Verification items for the finished model (mm, model axes). Face numbers are marked on the shaded views. A direction names the side the tool comes from. Give positions to 0.01 mm unless a question says otherwise; leave off trailing zeros. Write each loop counter-clockwise with the first axis right and the second up, starting at its lowest first coordinate (ties: lowest second). Pieces come first, ordered by that corner, then holes. Notation, with made-up numbers: M 12,-27 L 52,-27 A13 ccw 52,-4 Z; hole C 5,-39.5 d4. An arc over 180 degrees is marked long. Write item = value, one per line.
from build123d import *

# Parameters (mm, degrees)
F1_DEPTH = 4
F2_R     = 2
F2_R_2   = 3.5
F3_DEPTH = 25
F4_R     = 4.99999


# Not quite as in the source:
# - a fillet or chamfer is up to 0.001 mm smaller than in the source, because OpenCascade refuses the exact size


with BuildPart() as f1:
    # F0 (on Top) → F1 (new body)
    with BuildSketch(Plane.XY):
        Polygon((-5, 65), (-5, 0), (-30, 0), (-30, -14), (30, -14), (30, 0), (5, 0), (5, 65), align=None)
    extrude(amount=F1_DEPTH)

    # F2 (on face) → F3 (cut)
    with BuildSketch(Plane.XY.offset(4)):
        with Locations((-25, -7)):
            Circle(F2_R)
        with Locations((25, -7)):
            Circle(F2_R)
        with Locations((0, -7)):
            Circle(F2_R_2)
        with Locations((0, 61)):
            Circle(F2_R)
    extrude(amount=-F3_DEPTH, mode=Mode.SUBTRACT)

    # F4 (radius 5 in the source; OpenCascade refuses exactly that, so slightly less here)
    f4_edges = [f1.edges().sort_by_distance(p)[0] for p in [
        (-30, -14, 2),
        (-30, 0, 2),
        (30, -14, 2),
        (30, 0, 2),
        (5, 65, 2),
        (-5, 65, 2),
    ]]
    fillet(f4_edges, radius=F4_R)


solid = f1.part
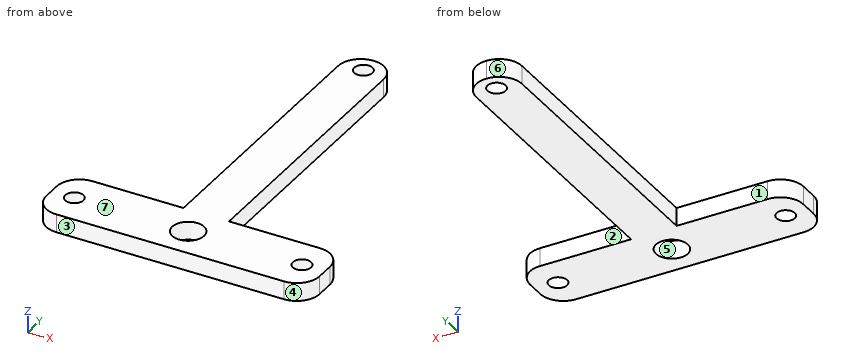
1) Cross-section at A-A on y = -7. Record the boundary of the cut face in (x, z), plus the area to 3 significant figures.
From the geometry:
outline = M -30,0 L -27,0 L -27,4 L -30,4 Z; M -23,0 L -3.5,0 L -3.5,4 L -23,4 Z; M 3.5,0 L 23,0 L 23,4 L 3.5,4 Z; M 27,0 L 30,0 L 30,4 L 27,4 Z
area = 180 mm^2
2) Draft check along X on the marked faces 4, 5, 6 and 7. Enter one of: +X half, -X half, draft (parallel to the pull), parting line (faces both ways), or undercut.
From the geometry:
face_4 = +X half
face_5 = undercut
face_6 = -X half
face_7 = draft
3) Cross-section at B-B on z = 1.6. Count the separate pieces of the cut face and the enclosed holes in it, plus the area to 3 significant figures.
From the geometry:
separate_pieces = 1
enclosed_holes = 4
area = 1,380 mm^2
4) Material ranges on probe 1 along Y at (x, z) = (0, 1.65); probe 2 along Y at (x, z) = (-25, 1.8); probe 3 along Y at (x, z) = (-0.5, 0.65), recorded low to high. Write a range as from..to.
From the geometry:
probe_1 = -14..-10.5, -3.5..59, 63..65
probe_2 = -14..-9, -5..0
probe_3 = -14..-10.46, -3.54..59.06, 62.94..64.97
5) Cross-section at C-C on y = 61. Record the boundary of the cut face in (x, z).
From the geometry:
outline = M -4.9,0 L -2,0 L -2,4 L -4.9,4 Z; M 2,0 L 4.9,0 L 4.9,4 L 2,4 Z
6) Tool access check on the marked faces 1, 2 and 3. Record the directions out of +Z, -Z, +X, -X, +Y, -Y that give a thin tool (end or side, any length) a straight path to the whole face; none if there is none.
From the geometry:
face_1 = +Z, -Z, -X, +Y
face_2 = +Z, -Z, +X, +Y
face_3 = +Z, -Z, +X, -X, -Y
7) Depth check by flat-ended pin: P1, Ø2, axis at x = -13, z = 2.5, coming from the +Y side; P2, Ø1, axis at y = 48, z = 3, coming from the +X side; P3, Ø1.5, axis at y = -0.5, z = 3.5, coming from the +X side. Enter the tip coordinate at first touch or a pass-through.
From the geometry:
P1 = 0
P2 = 5
P3 = 28.31
8) Cross-section at D-D on x = -13. Record the boundary of the cut face in (y, z), plus the area to 3 significant figures.
From the geometry:
outline = M -14,0 L 0,0 L 0,4 L -14,4 Z
area = 56.0 mm^2
